The listing builds one solid part. Answer for the finished solid, in the listing's coordinates (mm). Face numbers are marked on the shaded views. Coordinates: 2 decimals unless noted, no trailing zeros. Order: outer loops, then holes, each group sorted by start corner. A loop starts at its lowest first (then second) coordinate and runs counter-clockwise, first axis right, second up. Notation, with made-up numbers: (25, 76) -> (83, 76) arc R11 ccw to (83, 92) -> close; hole circle Ø4 at (30, 77). An arc over 180 degrees is marked (long way). Write item = value, one per line.
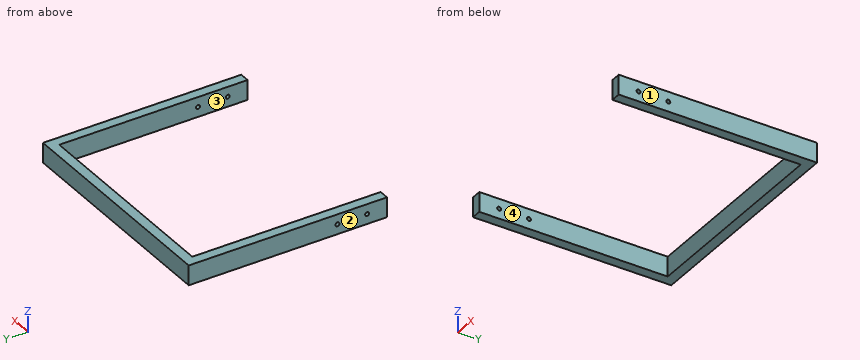
from build123d import *

# Parameters (mm, degrees)
BOSS_EXTRUDE1_DEPTH = 10
SKETCH2_R           = 2
CUT_EXTRUDE1_DEPTH  = 305.95901364


with BuildPart() as part:
    # Sketch1 → Boss-Extrude1 (new, symmetric)
    with BuildSketch(Plane.XY):
        Polygon((0, 0), (0, 200), (230, 200), (230, 0), (220, 0), (220, 190), (10, 190), (10, 0), align=None)
    extrude(amount=BOSS_EXTRUDE1_DEPTH, both=True)

    # Sketch2 → Cut-Extrude1 (cut, through all)
    with BuildSketch(Plane.ZY):
        with Locations((0, 20)):
            Circle(SKETCH2_R)
        with Locations((0, 50)):
            Circle(SKETCH2_R)
    extrude(amount=-CUT_EXTRUDE1_DEPTH, mode=Mode.SUBTRACT)


solid = part.part
Q1. Each of these flat-tipped pins is pushed along its axis until it touches: pin 1 Ø2.5 at (y, z) = (20, 0) entering from +X; pin 2 Ø1 at (y, z) = (126.5, 3) entering from -X; pin 3 Ø2 at (x, z) = (60.5, -2) entering from -Y. Where does it stop, or does it pass through?
The answers:
pin_1 = through
pin_2 = 0
pin_3 = 190
Q2. Find the intervals of material crossed by line 1 along Y through (x, z) = (5.5, 0); line 2 along X through (y, z) = (123, 6.5); line 3 along Y through (x, z) = (210.5, 8.25), in increasing order.
The answers:
line_1 = 0 to 18, 22 to 48, 52 to 200
line_2 = 0 to 10, 220 to 230
line_3 = 190 to 200
Q3. The mould has two halves that part along X. Classify the marked faces 1, 2, 3 and 4: released by +X, released by -X, zero draft, split by the parting line, or undercut.
The answers:
face_1 = released by +X
face_2 = released by -X
face_3 = undercut
face_4 = undercut
Q4. Section A-A, the plane y = 180.5 is taken. Give the vertices of the cut face in (x, z).
The answers:
outline = (0, -10) -> (10, -10) -> (10, 10) -> (0, 10) -> close; (220, -10) -> (230, -10) -> (230, 10) -> (220, 10) -> close
Q5. Section C-C, the plane x = 115 is taken. Give the vertices of the cut face in (y, z).
The answers:
outline = (190, -10) -> (200, -10) -> (200, 10) -> (190, 10) -> close
Q6. Section B-B, the plane z = -7 is taken. Give the vertices of the cut face in (x, y), plus the area to 3 significant figures.
The answers:
outline = (0, 0) -> (10, 0) -> (10, 190) -> (220, 190) -> (220, 0) -> (230, 0) -> (230, 200) -> (0, 200) -> close
area = 6,100 mm2
